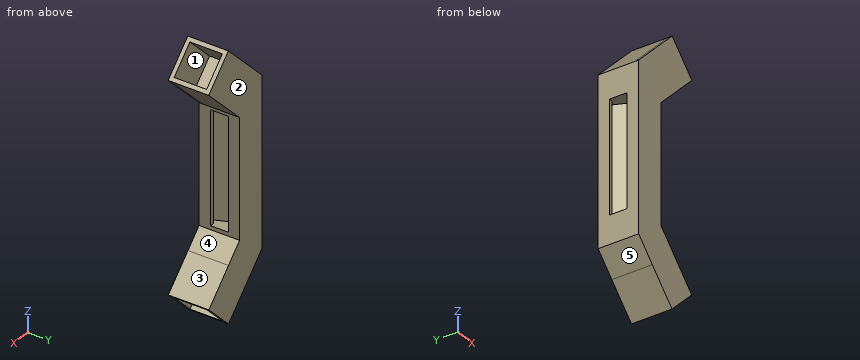
from build123d import *

# Parameters (mm, degrees)
EXTRUDE_1_DEPTH          = 2.5
EXTRUDE_2_DEPTH          = 20.2
EXTRUDE_3_DEPTH          = 2.5
CUT_EXTRUDE_1_DEPTH      = 35
CUT_EXTRUDE_1_DEPTH_BACK = 35


with BuildPart() as part:
    # 스케치1 → 보스-돌출1 (new body)
    with BuildSketch(Plane(origin=(0, 0, 0), x_dir=(1, 0, 0), z_dir=(0, 1, 0))):
        Polygon((-40.78505036, -82.204604484), (-58.462719889, -64.526934954), (-70.873239565, -52.116415278), (-70.873239565, 52.78521642), (-58.606071899, 65.106091447), (-40.92840237, 82.783760977), (-23.25073284, 65.106091447), (-40.92391218, 47.432912107), (-50.873239565, 37.425795029), (-50.873239565, -36.761076219), (-40.78505036, -46.849265425), (-23.10738083, -64.526934954), align=None)
    extrude(amount=EXTRUDE_1_DEPTH)

    # 스케치2 → 보스-돌출2 (add)
    with BuildSketch(Plane(origin=(0, 2.5, 0), x_dir=(1, 0, 0), z_dir=(0, 1, 0))):
        Polygon((-25.018499793, 66.8738584), (-42.694238669, 49.198119524), (-56.836374293, 63.340255148), (-39.160635417, 81.015994024), (-40.92840237, 82.783760977), (-58.606071899, 65.106091447), (-70.873239565, 52.78521642), (-70.873239565, -52.116415278), (-40.78505036, -82.204604484), (-39.017283407, -80.436837531), (-56.694952937, -62.759168001), (-42.552817313, -48.617032378), (-24.875147783, -66.294701907), (-23.10738083, -64.526934954), (-50.873239565, -36.761076219), (-50.873239565, 37.425795029), (-40.92391218, 47.432912107), (-23.25073284, 65.106091447), align=None)
    extrude(amount=EXTRUDE_2_DEPTH)

    # 스케치3 → 보스-돌출3 (add)
    with BuildSketch(Plane(origin=(0, 22.7, 0), x_dir=(1, 0, 0), z_dir=(0, 1, 0))):
        Polygon((-40.78505036, -82.204604484), (-23.10738083, -64.526934954), (-50.873239565, -36.761076219), (-50.873239565, 37.425795029), (-40.92391218, 47.432912107), (-23.25073284, 65.106091447), (-40.92840237, 82.783760977), (-58.606071899, 65.106091447), (-70.873239565, 52.78521642), (-70.873239565, -52.116415278), align=None)
    extrude(amount=EXTRUDE_3_DEPTH)

    # 스케치4 → 컷-돌출1 (cut, two sides: drawn at the far end of the back side and taken through both)
    with BuildSketch(Plane.XY.offset(-CUT_EXTRUDE_1_DEPTH_BACK)):
        Polygon((-50.873239565, 18.2), (-50.873239565, 16.507811734), (-50.873239565, 8.892188266), (-50.873239565, 7.2), (-53.373239565, 7.2), (-53.373239565, 2.2), (-54.873239565, 2.2), (-59.373239565, 12.7), (-54.873239565, 23.2), (-53.373239565, 23.2), (-53.373239565, 18.2), align=None)
        Polygon((-70.873239565, 18.2), (-68.373239565, 18.2), (-68.373239565, 23.2), (-66.873239565, 23.2), (-62.373239565, 12.7), (-66.873239565, 2.2), (-68.373239565, 2.2), (-68.373239565, 7.2), (-70.873239565, 7.2), align=None)
    extrude(amount=CUT_EXTRUDE_1_DEPTH + CUT_EXTRUDE_1_DEPTH_BACK, mode=Mode.SUBTRACT)


solid = part.part
Verification items for the finished model (mm, model axes). Face numbers are marked on the shaded views. A direction names the side the tool comes from. Round coordinates to 2 decimals unless told otherwise and drop trailing zeros. Loops run counter-clockwise (first coordinate to the right, second up) from the corner with the lowest first, then second, coordinate; pieces in that order, holes last. Notation, with made-up numbers: (40, -37) - (79, -37) arc R8 cw to (79, -28) - close; hole circle Ø7 at (-32, 66). An arc over 180 degrees is marked (long way). Answer in a Markdown table with one row per item. Add a question column.
Q1. Section check B-B on z = -7. Enter the section's corners in (x, y), plus the area to 4 significant figures.
Q2. Section check D-D on y = 5. Enter the section's corners in (x, z).
Q3. Release check for a two-part mould opening along Y. For the marked faces 1, 2 and 3 record: pulls with the +Y half, pulls with the -Y half, needs draft (parallel to the pull), parting line crosses it, or undercut.
Q4. Section check A-A on x = -46.5. Enter the section's corners in (y, z).
Q5. Tool access check on the marked faces 4 and 5. Record the directions out of +Z, -Z, +X, -X, +Y, -Y that give a thin tool (end or side, any length) a straight path to the whole face; none if there is none.
Q6. Material ranges on line 1 (X direction, y = 19, z = 17.5); line 2 (Z direction, x = -40, y = 5.75); line 3 (Y direction, x = -35.5, z = 65), recorded low to high.
Q7. Section check C-C on x = -37. Enter the section's corners in (y, z).
Q8. Gauge pin test, flat ends, axial feed: pin 1 (2 mm diameter, centred on x = -52.5, z = 1, fed in from -Y); pin 2 (2 mm diameter, centred on x = -61.5, y = 10.5, fed in from +Z); pin 3 (4 mm diameter, centred on y = 14.5, z = -50, fed in from +X); pin 4 (5 mm diameter, centred on y = 12.5, z = -6.5, fed in from -X). Record the tip position at first contact, or that the pin passes through.
Found:
| question | item | result |
|---|---|---|
| 1 | outline | (-70.87, 0) - (-50.87, 0) - (-50.87, 7.2) - (-53.37, 7.2) - (-53.37, 2.2) - (-54.87, 2.2) - (-59.37, 12.7) - (-54.87, 23.2) - (-53.37, 23.2) - (-53.37, 18.2) - (-50.87, 18.2) - (-50.87, 25.2) - (-70.87, 25.2) - (-70.87, 18.2) - (-68.37, 18.2) - (-68.37, 23.2) - (-66.87, 23.2) - (-62.37, 12.7) - (-66.87, 2.2) - (-68.37, 2.2) - (-68.37, 7.2) - (-70.87, 7.2) - close |
| 1 | area | 291.5 mm² |
| 2 | outline | (-70.87, -52.79) - (-58.61, -65.11) - (-40.93, -82.78) - (-39.16, -81.02) - (-56.84, -63.34) - (-42.69, -49.2) - (-25.02, -66.87) - (-23.25, -65.11) - (-40.92, -47.43) - (-50.87, -37.43) - (-50.87, 36.76) - (-23.11, 64.53) - (-24.88, 66.29) - (-42.55, 48.62) - (-56.69, 62.76) - (-39.02, 80.44) - (-40.79, 82.2) - (-70.87, 52.12) - close; hole (-68.37, -35) - (-65.67, -35) - (-65.67, 35) - (-68.37, 35) - close; hole (-56.07, -35) - (-53.37, -35) - (-53.37, 35) - (-56.07, 35) - close |
| 3 | face 1 | undercut |
| 3 | face 2 | pulls with the +Y half |
| 3 | face 3 | needs draft |
| 4 | outline | (0, -77.21) - (25.2, -77.21) - (25.2, -41.82) - (0, -41.82) - close; (0, 41.13) - (25.2, 41.13) - (25.2, 76.49) - (0, 76.49) - close; hole (2.5, -73.68) - (22.7, -73.68) - (22.7, -53) - (2.5, -53) - close; hole (2.5, 52.56) - (22.7, 52.56) - (22.7, 72.95) - (2.5, 72.95) - close |
| 5 | face 4 | +X, +Y, -Y |
| 5 | face 5 | -Z, -X, +Y, -Y |
| 6 | line 1 | x = -70.87 to -68.37, -65.07 to -56.67, -53.37 to -50.87 |
| 6 | line 2 | z = -81.86 to -80.18, -51.89 to -48.36, 47.63 to 51.17, 79.45 to 81.42 |
| 6 | line 3 | y = 0 to 2.5, 22.7 to 25.2 |
| 7 | outline | (0, -78.86) - (2.5, -78.86) - (2.5, -54.89) - (22.7, -54.89) - (22.7, -78.86) - (25.2, -78.86) - (25.2, -51.36) - (0, -51.36) - close; (0, 50.63) - (25.2, 50.63) - (25.2, 78.42) - (22.7, 78.42) - (22.7, 54.17) - (2.5, 54.17) - (2.5, 78.42) - (0, 78.42) - close |
| 8 | pin 1 | stops at y = 0 |
| 8 | pin 2 | stops at z = 62.49 |
| 8 | pin 3 | stops at x = -36.36 |
| 8 | pin 4 | stops at x = -63.53 |
